The listing builds one solid part. Answer for the finished solid, in the listing's coordinates (mm). Face numbers are marked on the shaded views. A direction names the side the tool comes from. Round coordinates to 2 decimals unless told otherwise and drop trailing zeros. Write each loop counter-clockwise with the first axis right and the second up, starting at its lowest first coordinate (ties: lowest second). Pieces come first, ordered by that corner, then holes.
Item 1: Find section C-C on y = -6.5. Give the vertices of the cut face in (x, z).
Item 2: A tool of negligible diameter and unlimited length cuts with its end or side. For the marked faces 1, 2 and 3, from which of +Z, -Z, +X, -X, +Y, -Y can it reach the whole face along a straight path? Write none if from no direction.
Item 3: Find section D-D on x = 90. Give the vertices of the cut face in (y, z).
Item 4: Find the intervals of material crossed by probe 1 along Y at (x, z) = (90, 4.25); probe 2 along Z at (x, y) = (5.75, -15); probe 3 along X at (y, z) = (-21.25, 93), in increasing order.
Item 5: Find section A-A on z = 90. Give the vertices of the cut face in (x, y).
Item 6: Each of these flat-tipped pins is pushed along its axis until it touches: pin 1 (5 mm diameter, centred on x = 61, y = -13.5, fed in from +Z); pin 2 (3 mm diameter, centred on y = -20.5, z = 45, fed in from +X); pin 3 (10 mm diameter, centred on x = 81, y = -6, fed in from +Z). Where does it stop, or does it pass through?
Item 7: Find section B-B on y = -15. Give the vertices of the cut face in (x, z), then the cut area to 3 significant figures.
Item 8: For a pull along X with two mould halves and no side action, classify the marked faces 4, 5, 6 and 7 as +X half, -X half, draft (parallel to the pull), parting line (faces both ways), or undercut.
```python
from build123d import *

# Parameters (mm, degrees)
F1_DEPTH = 30
F3_D     = 9
F3_DEPTH = 8.001
F5_D     = 9
F5_DEPTH = 8.001


with BuildPart() as f1:
    # F0 (on Front) → F1 (new body)
    with BuildSketch(Plane.XZ):
        Polygon((0, 100), (0, 0), (100, 0), (100, 8), (80, 8), (8, 80), (8, 100), align=None)
        Polygon((8, 8), (8, 68.686291501), (68.686291501, 8), align=None, mode=Mode.SUBTRACT)
    extrude(amount=F1_DEPTH)

    # F3 (through all, one way)
    with BuildSketch(Plane.XY.offset(8)):
        with Locations((35, -15), (90, -15)):
            Circle(F3_D / 2)
    extrude(amount=-F3_DEPTH, mode=Mode.SUBTRACT)

    # F5 (through all, one way)
    with BuildSketch(Plane.YZ.offset(8)):
        with Locations((-15, 90), (-15, 35)):
            Circle(F5_D / 2)
    extrude(amount=-F5_DEPTH, mode=Mode.SUBTRACT)


solid = f1.part
```
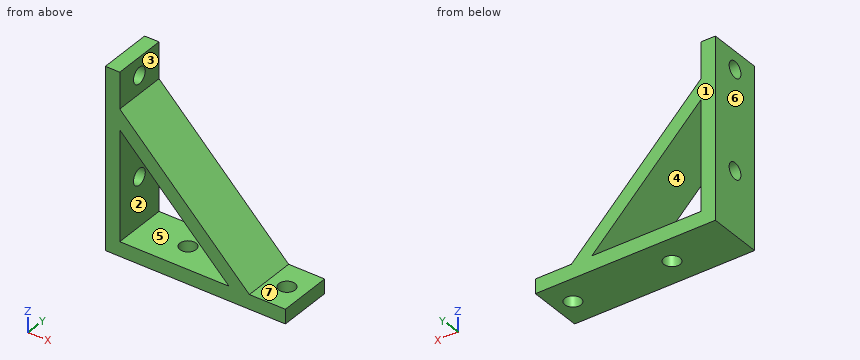
Check values:
1. outline: (0, 0) - (100, 0) - (100, 8) - (80, 8) - (8, 80) - (8, 100) - (0, 100) - close; hole (8, 8) - (68.69, 8) - (8, 68.69) - close
2. face 1: +Z, -Z, +X, -X, +Y
2. face 2: +Y, -Y
2. face 3: +Z, +X, +Y, -Y
3. outline: (-30, 0) - (-19.5, 0) - (-19.5, 8) - (-30, 8) - close; (-10.5, 0) - (0, 0) - (0, 8) - (-10.5, 8) - close
4. probe 1: y = -30 to -19.5, -10.5 to 0
4. probe 2: z = 0 to 30.5, 39.5 to 85.5, 94.5 to 100
4. probe 3: x = 0 to 8
5. outline: (0, -30) - (8, -30) - (8, -19.5) - (0, -19.5) - close; (0, -10.5) - (8, -10.5) - (8, 0) - (0, 0) - close
6. pin 1: stops at z = 29.5
6. pin 2: stops at x = 44.5
6. pin 3: stops at z = 12
7. outline: (0, 0) - (30.5, 0) - (30.5, 8) - (8, 8) - (8, 30.5) - (0, 30.5) - close; (0, 39.5) - (8, 39.5) - (8, 68.69) - (68.69, 8) - (39.5, 8) - (39.5, 0) - (85.5, 0) - (85.5, 8) - (80, 8) - (8, 80) - (8, 85.5) - (0, 85.5) - close; (0, 94.5) - (8, 94.5) - (8, 100) - (0, 100) - close; (94.5, 0) - (100, 0) - (100, 8) - (94.5, 8) - close
7. area: 2,000 mm2
8. face 4: undercut
8. face 5: undercut
8. face 6: -X half
8. face 7: draft
